Geometry check sheet. Reference: the model listing, model coordinates, mm. A direction names the side the tool comes from. Coordinates: 2 decimals unless noted, no trailing zeros. Order: outer loops, then holes, each group sorted by start corner. A loop starts at its lowest first (then second) coordinate and runs counter-clockwise, first axis right, second up. Notation, with made-up numbers: (-6, 78.5) - (1, 78.5) arc R22 ccw to (1, 84.5) - close; hole circle Ø2 at (15, -29). An arc over 180 degrees is marked (long way). Return JSON: item names as keys, results as strings. Group by question number.
Item 1: Section check A-A on x = -104. Enter the section's corners in (y, z), then the cut area to 3 significant figures.
Item 2: Tool access check on faces 1 (the flat face through (-115.807, 11.796, 0.07)), 2 (the flat face through (-110.534, 3.364, 0.07)), 3 (the flat face through (-95.164, 0.396, 0.07)), 4 (the cylindrical face through (-114.626, 5.693, 0.07)), 5 (the flat face through (-110.232, 18, 0)). Record the directions out of +Z, -Z, +X, -X, +Y, -Y that give a thin tool (end or side, any length) a straight path to the whole face; none if there is none.
Item 3: Section check C-C on x = -98. Enter the section's corners in (y, z), then the cut area to 3 significant figures.
Item 4: Draft check along Y on faces 6 (the flat face through (-111.285, 16.464, 0.07)), 7 (the flat face through (-116.763, 13.138, 0.07)), 8 (the flat face through (-114.36, 14.47, 0.07)), 9 (the cylindrical face through (-114, 2.28, 0.07)). Enter one of: pulls with the +Y half, pulls with the -Y half, needs draft (parallel to the pull), parting line crosses it, or undercut.
Item 5: Gauge pin test, flat ends, axial feed: pin 1 (0.6 mm diameter, centred on x = -101.5, z = 2, fed in from +Y); pin 2 (2 mm diameter, centred on x = -99, z = 1.5, fed in from -Y); pin 3 (1 mm diameter, centred on x = -98.5, z = 1, fed in from +Y). Record the tip position at first contact, or that the pin passes through.
Item 6: Scan lines: probe 1 along X at (y, z) = (14.5, -0.5); probe 2 along Y at (x, z) = (-114.5, 4.75); probe 3 along X at (y, z) = (11.25, -1). Record each from-to range of solid material in increasing order.
Item 7: Section check B-B on y = 10.5. Enter the section's corners in (x, z).
Item 8: Section check D-D on y = -6.75. Enter the section's corners in (x, z).
from build123d import *

# Parameters (mm, degrees)
SKETCH7_R           = 2.718976156
BOSS_EXTRUDE5_DEPTH = 5


with BuildPart() as part:
    # Sketch7 → Boss-Extrude5 (new body, symmetric)
    with BuildSketch(Plane.XY):
        with BuildLine():
            Line((-108.314342925, 18.989771489), (-110.232079527, 18.989771489))
            Line((-110.232079527, 18.989771489), (-110.232079527, 16.794247959))
            Line((-110.232079527, 16.794247959), (-112.368671741, 16.124256422))
            Line((-112.368671741, 16.124256422), (-112.848780488, 18.148130182))
            Line((-112.848780488, 18.148130182), (-114.689202025, 17.136193302))
            Line((-114.689202025, 17.136193302), (-113.802244367, 15.156219029))
            Line((-113.802244367, 15.156219029), (-114.926218754, 13.769061439))
            Line((-114.926218754, 13.769061439), (-116.638184972, 15.156219029))
            Line((-116.638184972, 15.156219029), (-117.890010894, 13.611272945))
            Line((-117.890010894, 13.611272945), (-115.604979487, 12.652206929))
            Line((-115.604979487, 12.652206929), (-116.014015282, 10.916483695))
            Line((-116.014015282, 10.916483695), (-117.890010894, 10.916483695))
            Line((-117.890010894, 10.916483695), (-117.890010894, 9.290502395))
            Line((-117.890010894, 9.290502395), (-116.103879087, 9.290502395))
            ThreePointArc((-116.103879087, 9.290502395), (-115.994870907, 8.589969318), (-115.814214218, 7.904409303))
            Line((-115.814214218, 7.904409303), (-117.890010894, 7.24106602))
            ThreePointArc((-117.890010894, 7.24106602), (-117.56834444, 6.386019614), (-117.162078542, 5.567776566))
            Line((-117.162078542, 5.567776566), (-115.261641584, 6.634217149))
            ThreePointArc((-115.261641584, 6.634217149), (-114.615525484, 5.680316792), (-113.819022014, 4.847866116))
            Line((-113.819022014, 4.847866116), (-115.261641584, 3.214524472))
            ThreePointArc((-115.261641584, 3.214524472), (-113.978252901, 2.268462787), (-112.548700742, 1.562417569))
            Line((-112.548700742, 1.562417569), (-111.759631654, 3.593753614))
            Line((-111.759631654, 3.593753614), (-109.273211226, 3.127790889))
            Line((-109.273211226, 3.127790889), (-109.273211226, 0.948580907))
            ThreePointArc((-109.273211226, 0.948580907), (-107.630782877, 1.098932073), (-106.042950797, 1.544987721))
            Line((-106.042950797, 1.544987721), (-106.785965128, 3.488554168))
            Line((-106.785965128, 3.488554168), (-91.16192211, -9.89798132))
            Line((-91.16192211, -9.89798132), (-87.560983072, -6.260758332))
            Line((-87.560983072, -6.260758332), (-102.982615742, 7.24106602))
            Line((-102.982615742, 7.24106602), (-102.732208234, 7.904409303))
            Line((-102.732208234, 7.904409303), (-100.286956522, 7.904409303))
            Line((-100.286956522, 7.904409303), (-100.286956522, 9.994657565))
            Line((-100.286956522, 9.994657565), (-102.40634455, 9.994657565))
            ThreePointArc((-102.40634455, 9.994657565), (-102.470378556, 10.930245938), (-102.661286329, 11.848385459))
            Line((-102.661286329, 11.848385459), (-100.710110893, 13.132180531))
            Line((-100.710110893, 13.132180531), (-101.856516581, 14.874544766))
            Line((-101.856516581, 14.874544766), (-103.536684982, 13.769061439))
            Line((-103.536684982, 13.769061439), (-104.442004457, 14.874544766))
            Line((-104.442004457, 14.874544766), (-102.908814063, 16.423183965))
            Line((-102.908814063, 16.423183965), (-105.01782302, 17.977337199))
            Line((-105.01782302, 17.977337199), (-106.042950797, 16.054300748))
            Line((-106.042950797, 16.054300748), (-108.314342925, 16.794247959))
            Line((-108.314342925, 16.794247959), (-108.314342925, 18.989771489))
        make_face()
        with Locations((-109.273211226, 9.994657565)):
            Circle(SKETCH7_R, mode=Mode.SUBTRACT)
    extrude(amount=BOSS_EXTRUDE5_DEPTH, both=True)


solid = part.part
Computed:
{
 "1": {"outline": "(1.1, -5) - (14.33, -5) - (14.33, 5) - (1.1, 5) - close; (15.32, -5) - (17.23, -5) - (17.23, 5) - (15.32, 5) - close", "area": "151 mm²"},
 "2": {"face 1": "+Z, -Z, -X", "face 2": "+Z, -Z, -Y", "face 3": "+Z, -Z, +X", "face 4": "+Z, -Z", "face 5": "+Z, -Z, +Y"},
 "3": {"outline": "(-4.04, -5) - (2.88, -5) - (2.88, 5) - (-4.04, 5) - close", "area": "69.2 mm²"},
 "4": {"face 6": "pulls with the +Y half", "face 7": "undercut", "face 8": "undercut", "face 9": "pulls with the -Y half"},
 "5": {"pin 1": "stops at y = 14.79", "pin 2": "stops at y = -4.04", "pin 3": "stops at y = 3.75"},
 "6": {"probe 1": "x = -117.17 to -115.83, -114.33 to -104.14, -102.43 to -101.61", "probe 2": "y = 2.61 to 4.08, 5.54 to 14.3, 16.71 to 17.24", "probe 3": "x = -115.94 to -111.69, -106.86 to -102.52"},
 "7": {"outline": "(-117.89, -5) - (-111.94, -5) - (-111.94, 5) - (-117.89, 5) - close; (-106.6, -5) - (-102.42, -5) - (-102.42, 5) - (-106.6, 5) - close"},
 "8": {"outline": "(-94.84, -5) - (-88.05, -5) - (-88.05, 5) - (-94.84, 5) - close"}
}
